from build123d import *

# Parameters (mm, degrees)
TROU_TARAUD_0_801_D = 5


with BuildPart() as part:
    # Esquisse1 → Révolution1 (revolve)
    with BuildSketch(Plane.XY, mode=Mode.PRIVATE) as r_volution1_sk:
        Polygon((-4.25, 5.769230769), (-5.25, 5.769230769), (-5.25, -11.328656218), (0, -11.328656218), (0, -10.328656218), (-4.25, -10.328656218), align=None)
    revolve(r_volution1_sk.sketch.rotate(Axis((0, 8.346153846, 0), (0, -1, 0)), 270), axis=Axis((0, 8.346153846, 0), (0, -1, 0)))

    # Trou taraudé #0-801 (through all)
    with Locations(Plane(origin=(-0.143240146, -3.686819395, 5.248045566), x_dir=(0.999627726819, 0, 0.027283837244), z_dir=(-0.027283837244, 0, 0.999627726819))):
        with Locations((0, 0)):
            Hole(TROU_TARAUD_0_801_D / 2)


solid = part.part
Input: part model. Units: mm. Frame: model coordinates. A direction names the side the tool comes from. Coordinates: 2 decimals unless noted, no trailing zeros. Loops run counter-clockwise (first coordinate to the right, second up) from the corner with the lowest first, then second, coordinate; pieces in that order, holes last. Notation, with made-up numbers: (18.25, -26) - (71.25, -26) arc R21 ccw to (71.25, 8) - close; hole circle Ø9 at (-18.5, 44.25). An arc over 180 degrees is marked (long way). Answer in a Markdown table with one row per item. Add a question column.
Item 1: Line query: line 1 along X through (y, z) = (-4.25, 0); line 2 along X through (y, z) = (-9, 1.75); line 3 along Z through (x, y) = (2, -1.25). Output: solid intervals per line, ascending. Write a range as [from, to].
Item 2: Contact query for flat-ended pins moving along their axis: P1, Ø3, axis at x = -2, z = 1.5, coming from the +Y side; P2, Ø2, axis at x = 0.5, y = -2.5, coming from the -Z side; P3, Ø6, axis at x = 1.5, y = -7, coming from the +Z side; P4, Ø1.5, axis at x = -2, y = -7.5, coming from the +Z side. Output: stop coordinate, or through.
Item 3: Mould query, pull axis Y, two halves, no side actions, for faces 1 (the flat face through (0, -10.329, 0)), 2 (the cylindrical face through (-1.225, -1.579, -4.394)), 3 (the flat face through (0, -11.329, 0)). Classes: released by +Y, released by -Y, zero draft, split by the parting line, or undercut.
Item 4: Section query A-A on y = -6. Return the cut outline in (x, z), then the cut area to 3 significant figures.
Item 5: Section query C-C on y = 0.75. Return the cut outline in (x, z), then the cut area to 3 significant figures.
Item 6: Section query B-B on z = 0. Return the cut outline in (x, y).
Item 7: Access query for faces 4 (the cylindrical face through (-1.46, -1.58, 4.29)), 5 (the cylindrical face through (2.59, -2.17, -3.37)), 6 (the cylindrical face through (-3.55, -2.9, -3.87)). Directions: +Z, -Z, +X, -X, +Y, -Y. A direction counts if a zero-diameter tool reaches every point of the face in a straight line with its end or side. Return the directions, or none.
Item 8: Section query D-D on x = 0. State how many separate pieces and enclosed holes the cut face has, then the cut area to 3 significant figures.
Recorded:
| question | item | result |
|---|---|---|
| 1 | line 1 | [-5.25, -4.25], [4.25, 5.25] |
| 1 | line 2 | [-4.95, -3.87], [3.87, 4.95] |
| 1 | line 3 | [-4.85, -3.75], [3.75, 4.85] |
| 2 | P1 | y = -10.33 |
| 2 | P2 | through |
| 2 | P3 | z = 5.25 |
| 2 | P4 | z = 5.1 |
| 3 | face 1 | released by +Y |
| 3 | face 2 | undercut |
| 3 | face 3 | released by -Y |
| 4 | outline | (-1.09, 5.14) arc R5.25 ccw to (-0.81, -5.19) - (-0.83, -4.17) arc R4.25 cw to (-1.06, 4.12) - close; (0.81, 5.19) - (0.83, 4.17) arc R4.25 cw to (1.06, -4.12) - (1.09, -5.14) arc R5.25 ccw to start |
| 4 | area | 26.0 mm^2 |
| 5 | outline | circle Ø10.5 at (0, 0); hole circle Ø8.5 at (0, 0) |
| 5 | area | 29.8 mm^2 |
| 6 | outline | (-5.25, -11.33) - (5.25, -11.33) - (5.25, 5.77) - (4.25, 5.77) - (4.25, -10.33) - (-4.25, -10.33) - (-4.25, 5.77) - (-5.25, 5.77) - close |
| 7 | face 4 | none |
| 7 | face 5 | +Y |
| 7 | face 6 | +Y, -Y |
| 8 | separate pieces | 3 |
| 8 | enclosed holes | 0 |
| 8 | area | 32.7 mm^2 |
